Could you check a few things on this model? Use its own coordinates, in mm. Face numbers are marked on the shaded views. Coordinates: 2 decimals unless noted, no trailing zeros. Write each loop counter-clockwise with the first axis right and the second up, starting at its lowest first coordinate (ties: lowest second). Pieces come first, ordered by that corner, then holes. Notation, with made-up numbers: M 16,65.25 L 22,65.25 A24 cw 22,85.25 Z; hole C 9,-8.75 d10. An arc over 180 degrees is marked long. Write item = value, one per line.
```python
from build123d import *

# Parameters (mm, degrees)
F1_DEPTH = 917.5
F2_DEPTH = 40


with BuildPart() as f1:
    # F0 (on Front) → F1 (new body)
    with BuildSketch(Plane.XZ):
        with BuildLine():
            ThreePointArc((-102.5, -13.5), (-101.767767, -15.267767), (-100, -16))
            Line((-100, -16), (100, -16))
            ThreePointArc((100, -16), (101.767767, -15.267767), (102.5, -13.5))
            Line((102.5, -13.5), (102.5, 0))
            Line((102.5, 0), (99.5, 0))
            Line((99.5, 0), (99.5, -10.5))
            ThreePointArc((99.5, -10.5), (98.767767, -12.267767), (97, -13))
            Line((97, -13), (-97, -13))
            ThreePointArc((-97, -13), (-98.767767, -12.267767), (-99.5, -10.5))
            Line((-99.5, -10.5), (-99.5, 0))
            Line((-99.5, 0), (-102.5, 0))
            Line((-102.5, 0), (-102.5, -13.5))
        make_face()
        with BuildLine():
            Line((-96.5, 0), (-99.5, 0))
            Line((-99.5, 0), (-99.5, -10.5))
            ThreePointArc((-99.5, -10.5), (-98.767767, -12.267767), (-97, -13))
            Line((-97, -13), (97, -13))
            ThreePointArc((97, -13), (98.767767, -12.267767), (99.5, -10.5))
            Line((99.5, -10.5), (99.5, 0))
            Line((99.5, 0), (96.5, 0))
            Line((96.5, 0), (96.5, -7.5))
            ThreePointArc((96.5, -7.5), (95.767767, -9.267767), (94, -10))
            Line((94, -10), (-94, -10))
            ThreePointArc((-94, -10), (-95.767767, -9.267767), (-96.5, -7.5))
            Line((-96.5, -7.5), (-96.5, 0))
        make_face()
    extrude(amount=F1_DEPTH)

    # F0 (on Front) → F2 (cut)
    with BuildSketch(Plane.XZ):
        with BuildLine():
            ThreePointArc((-102.5, -13.5), (-101.767767, -15.267767), (-100, -16))
            Line((-100, -16), (100, -16))
            ThreePointArc((100, -16), (101.767767, -15.267767), (102.5, -13.5))
            Line((102.5, -13.5), (102.5, 0))
            Line((102.5, 0), (99.5, 0))
            Line((99.5, 0), (99.5, -10.5))
            ThreePointArc((99.5, -10.5), (98.767767, -12.267767), (97, -13))
            Line((97, -13), (-97, -13))
            ThreePointArc((-97, -13), (-98.767767, -12.267767), (-99.5, -10.5))
            Line((-99.5, -10.5), (-99.5, 0))
            Line((-99.5, 0), (-102.5, 0))
            Line((-102.5, 0), (-102.5, -13.5))
        make_face()
    extrude(amount=F2_DEPTH, mode=Mode.SUBTRACT)


solid = f1.part
```
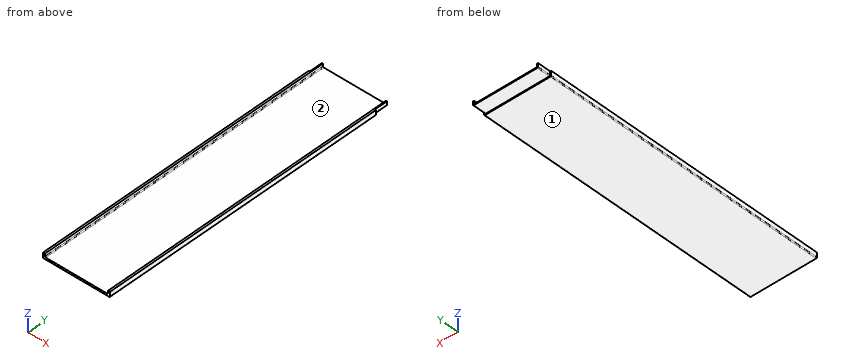
Item 1: Imagine slicing it at A-A (z = -2.5). Write out the boundary of the cut face in (x, y).
Numbers:
outline = M -102.5,-917.5 L -96.5,-917.5 L -96.5,0 L -99.5,0 L -99.5,-40 L -102.5,-40 Z; M 96.5,-917.5 L 102.5,-917.5 L 102.5,-40 L 99.5,-40 L 99.5,0 L 96.5,0 Z
Item 2: If I drill on line 1 along X through (y, z) = (-666.5, -0.75); line 2 along Z through (x, y) = (56, -92); line 3 along X through (y, z) = (-504.5, -14), over which ranges is the centre line in solid material (lowest first)?
Numbers:
line_1 = -102.5 to -96.5, 96.5 to 102.5
line_2 = -16 to -10
line_3 = -102.45 to 102.45
Item 3: If we mould it in two halves opening along X, with no side actions, what happens to the marked faces 1 and 2? For each: pulls with the +X half, pulls with the -X half, needs draft (parallel to the pull), parting line crosses it, or undercut.
Numbers:
face_1 = needs draft
face_2 = undercut
Item 4: Imagine slicing it at B-B (y = -403). Write out the boundary of the cut face in (x, z), and give its area (3 significant figures).
Numbers:
outline = M -102.5,-13.5 A2.5 ccw -100,-16 L 100,-16 A2.5 ccw 102.5,-13.5 L 102.5,0 L 96.5,0 L 96.5,-7.5 A2.5 cw 94,-10 L -94,-10 A2.5 cw -96.5,-7.5 L -96.5,0 L -102.5,0 Z
area = 1,350 mm²
Item 5: Imagine slicing it at C-C (x = 4.5). Write out the boundary of the cut face in (y, z).
Numbers:
outline = M -917.5,-16 L -40,-16 L -40,-13 L 0,-13 L 0,-10 L -917.5,-10 Z
Item 6: I'm going to push flat-ended pins straight in: P1, Ø5, axis at y = -12, z = -6.5, coming from the +X side; P2, Ø8.5, axis at y = -30, z = -3, coming from the -X side; P3, Ø20, axis at x = 4.5, y = -19, coming from the -Z side. Where does each tip first touch, or does it pass through?
Numbers:
P1 = 99.5
P2 = -99.5
P3 = -13
